Source: three-view drawing plus pictorial views. Frame: mm from the lowest corner of the part. A direction names the side the tool comes from. Give positions to 0.01 mm unless a question says otherwise; leave off trailing zeros. Loops run counter-clockwise (first coordinate to the right, second up) from the corner with the lowest first, then second, coordinate; pieces in that order, holes last. Notation, with made-up numbers: (74, -8.5) -> (111, -8.5) arc R25 cw to (111, 5.5) -> close; hole circle Ø9 at (-29.5, 35). An arc over 180 degrees is marked (long way). Answer as a JSON object with one key per item and string values. Group by question number.
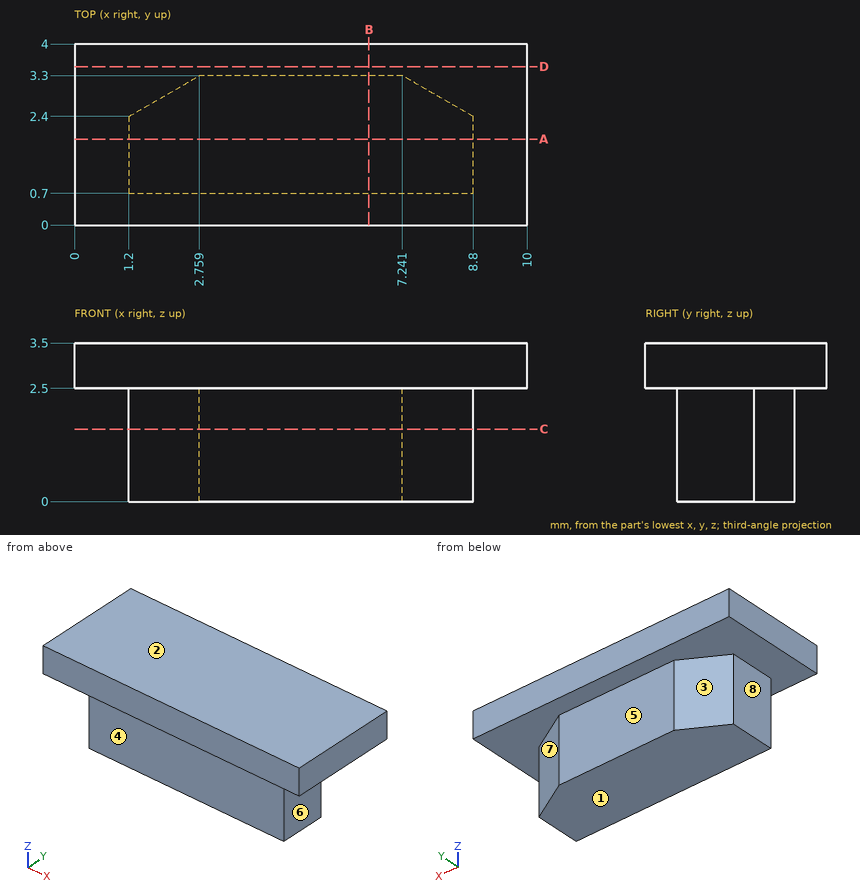
(1) Access query for the marked faces 4, 5, 6, 7 and 8. Directions: +Z, -Z, +X, -X, +Y, -Y. A direction counts if a zero-diameter tool reaches every point of the face in a straight line with its end or side. Return the directions, or none.
(2) Section query C-C on z = 1.6. Return the cut outline in (x, y), plus the area to 3 significant figures.
(3) Section query A-A on y = 1.9. Return the cut outline in (x, z), plus the area to 3 significant figures.
(4) Material intervals for line 1 (Z direction, x = 6, y = 0.25); line 2 (X direction, y = 2.05, z = 2); line 3 (Y direction, x = 4.5, z = 1.85), sorted ascending. Write a range as from..to.
(5) Section query B-B on x = 6.5. Return the cut outline in (y, z).
(6) Section query D-D on y = 3.5. Return the cut outline in (x, z), plus the area to 3 significant figures.
(7) First-contact query: pin 1 (1 mm diameter, centred on x = 3.5, y = 3, fed in from -Z); pin 2 (0.8 mm diameter, centred on y = 1.5, z = 1, fed in from -X); pin 3 (2 mm diameter, centred on x = 7, z = 1, fed in from -Y); pin 4 (0.5 mm diameter, centred on y = 1.5, z = 1, fed in from +X). Flat tips, straight axial feed; report the tip coordinate or a pass-through.
(8) Mould query, pull axis Z, two halves, no side actions, for the marked faces 1, 2 and 3. Classes: pulls with the +Z half, pulls with the -Z half, needs draft (parallel to the pull), parting line crosses it, or undercut.
Result:
{
 "1": {"face 4": "-Z, +X, -X, -Y", "face 5": "-Z, +X, -X, +Y", "face 6": "-Z, +X, +Y, -Y", "face 7": "-Z, +X, +Y", "face 8": "-Z, -X, +Y, -Y"},
 "2": {"outline": "(1.2, 0.7) -> (8.8, 0.7) -> (8.8, 2.4) -> (7.24, 3.3) -> (2.76, 3.3) -> (1.2, 2.4) -> close", "area": "18.4 mm²"},
 "3": {"outline": "(0, 2.5) -> (1.2, 2.5) -> (1.2, 0) -> (8.8, 0) -> (8.8, 2.5) -> (10, 2.5) -> (10, 3.5) -> (0, 3.5) -> close", "area": "29.0 mm²"},
 "4": {"line 1": "2.5..3.5", "line 2": "1.2..8.8", "line 3": "0.7..3.3"},
 "5": {"outline": "(0, 2.5) -> (0.7, 2.5) -> (0.7, 0) -> (3.3, 0) -> (3.3, 2.5) -> (4, 2.5) -> (4, 3.5) -> (0, 3.5) -> close"},
 "6": {"outline": "(0, 2.5) -> (10, 2.5) -> (10, 3.5) -> (0, 3.5) -> close", "area": "10.0 mm²"},
 "7": {"pin 1": "z = 0", "pin 2": "x = 1.2", "pin 3": "y = 0.7", "pin 4": "x = 8.8"},
 "8": {"face 1": "pulls with the -Z half", "face 2": "pulls with the +Z half", "face 3": "needs draft"}
}
